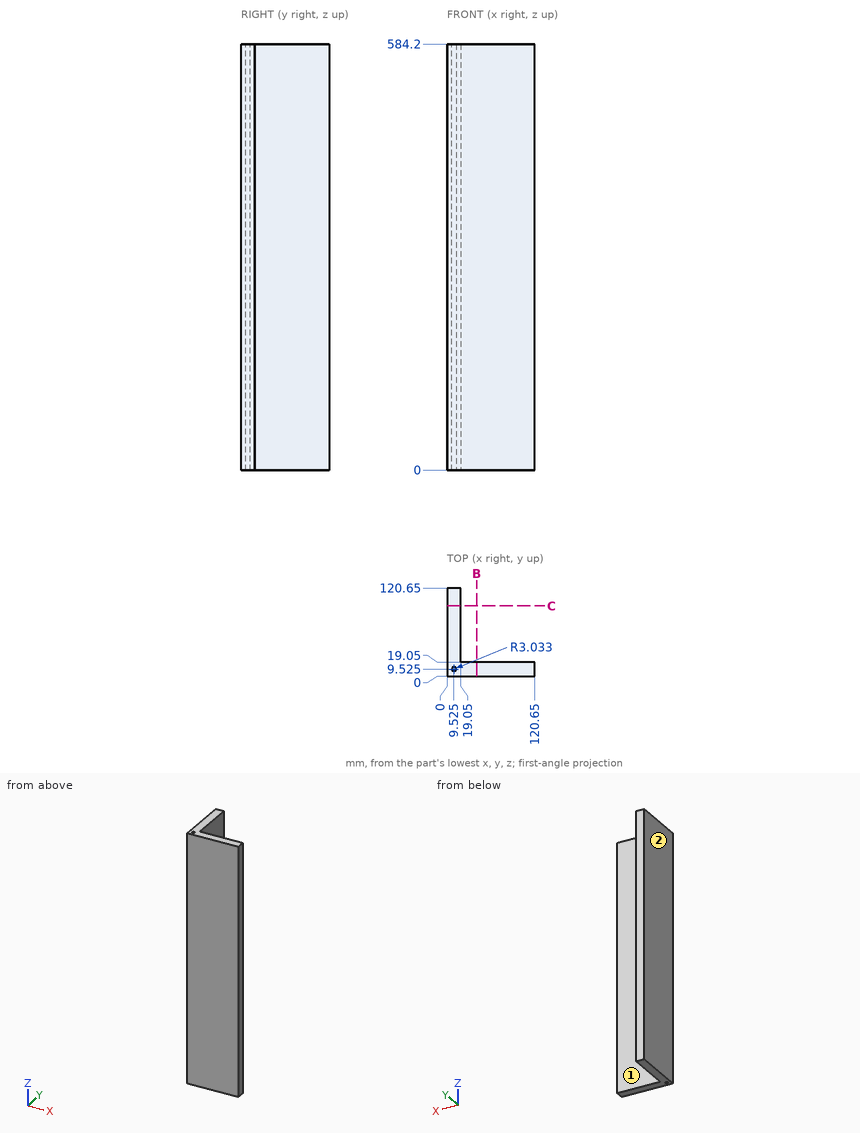
Could you check a few things on this drawing? It's one solid part, dimensions in mm from its lowest x, y, z. A direction names the side the tool comes from. Give positions to 0.01 mm unless a question says otherwise; leave off trailing zeros. Order: outer loops, then holes, each group sorted by start corner. A loop starts at its lowest first (then second) coordinate and runs counter-clockwise, first axis right, second up. Notation, with made-up numbers: (57, 5.5) - (95, 5.5) arc R33 ccw to (95, 33.5) - close; hole circle Ø2 at (17.5, 47). An arc over 180 degrees is marked (long way). One line per question, with ' | ' between items. Start each with the question number.
Item 1: I'm going to push a flat-ended pin straight in: pin 1 Ø3 at (y, z) = (81, 524.5) entering from +X. Where does the tip first touch, or does it pass through?
Item 2: I need wall thicknesses on probe 1 along Y at (x, z) = (7.5, 253.5); probe 2 along X at (y, z) = (9, 336); probe 3 along X at (y, z) = (74, 62). Which ranges of each line are inside material? Lowest first, please. Write a range as [from, to].
Item 3: I want a section at B-B on x = 40.5. Write out the boundary of the cut face in (y, z), then the cut area to 3 significant figures.
Item 4: For the marked faces 1 and 2, which set-ups out of +Z, -Z, +X, -X, +Y, -Y let a thin tool reach every point of the face, with its end or its side?
Verdict:
1) pin 1: x = 19.05
2) probe 1: [0, 7.27], [11.78, 120.65] | probe 2: [0, 6.54], [12.51, 120.65] | probe 3: [0, 19.05]
3) outline: (0, 0) - (19.05, 0) - (19.05, 584.2) - (0, 584.2) - close | area: 11,100 mm^2
4) face 1: +Z, -Z, +X, +Y | face 2: +Z, -Z, -X, +Y, -Y
